from build123d import *

# Parameters (mm, degrees)
BOSS_EXTRUDE1_DEPTH = 5.7
SKETCH2_R           = 14.85
CUT_EXTRUDE1_DEPTH  = 6.7


with BuildPart() as part:
    # Sketch1 → Boss-Extrude1 (new body)
    with BuildSketch(Plane.XY):
        Polygon((-159.83650641, 166.052929421), (-154.13650641, 166.052929421), (-154.13650641, 115.252929421), (-160.286019508, 115.252929421), (-160.286019508, 50.952929421), (-154.13650641, 50.952929421), (-154.13650641, 0.152929421), (-159.83650641, 0.152929421), (-159.83650641, -24.847070579), (444.06349359, -24.847070579), (444.06349359, 0.899402865), (438.36349359, 0.899402865), (438.36349359, 51.699402865), (444.06349359, 51.699402865), (444.06349359, 77.821679421), (-159.83650641, 191.052929421), align=None)
    extrude(amount=BOSS_EXTRUDE1_DEPTH)

    # Sketch2 → Cut-Extrude1 (cut, through all)
    with BuildSketch(Plane.XY.offset(5.7)):
        with Locations((317.523696403, 24.846574105)):
            Circle(SKETCH2_R)
        Polygon((287.261228118, 47.129406511), (288.311706475, 52.731771656), (238.381855706, 62.093929643), (237.331377349, 56.491564498), align=None)
        Polygon((177.179115935, 67.770488147), (178.229594292, 73.372853292), (128.299743522, 82.735011279), (127.249265166, 77.132646134), align=None)
        Polygon((-92.56491366, 124.199043845), (-41.76491366, 114.673727458), (-42.83369916, 108.973727458), (-93.63369916, 118.499043845), align=None)
        Polygon((18.217631339, 103.376092915), (68.147482108, 94.013934928), (67.097003751, 88.411569783), (17.167152982, 97.77372777), align=None)
        with BuildLine():
            Line((-24.756085794, 42.151529897), (-24.756085794, 36.301350189))
            ThreePointArc((-24.756085794, 36.301350189), (-25.048979012, 35.594243408), (-25.756085794, 35.301350189))
            Line((-25.756085794, 35.301350189), (-125.756085794, 35.301350189))
            ThreePointArc((-125.756085794, 35.301350189), (-126.463192575, 35.594243408), (-126.756085794, 36.301350189))
            Line((-126.756085794, 36.301350189), (-126.756085794, 42.151529897))
            ThreePointArc((-126.756085794, 42.151529897), (-126.463192575, 42.858636678), (-125.756085794, 43.151529897))
            Line((-125.756085794, 43.151529897), (-25.756085794, 43.151529897))
            ThreePointArc((-25.756085794, 43.151529897), (-25.048979012, 42.858636678), (-24.756085794, 42.151529897))
        make_face()
        Polygon((348.312558617, 41.531771968), (347.252926688, 35.880589395), (398.052926688, 26.355273008), (399.112558617, 32.006455581), align=None)
        with BuildLine():
            Line((-25.756085794, 56.60407475), (-125.756085794, 56.60407475))
            ThreePointArc((-125.756085794, 56.60407475), (-126.463192575, 56.311181531), (-126.756085794, 55.60407475))
            Line((-126.756085794, 55.60407475), (-126.756085794, 49.753895042))
            ThreePointArc((-126.756085794, 49.753895042), (-126.463192575, 49.046788261), (-125.756085794, 48.753895042))
            Line((-125.756085794, 48.753895042), (-25.756085794, 48.753895042))
            ThreePointArc((-25.756085794, 48.753895042), (-25.048979012, 49.046788261), (-24.756085794, 49.753895042))
            Line((-24.756085794, 49.753895042), (-24.756085794, 55.60407475))
            ThreePointArc((-24.756085794, 55.60407475), (-25.048979012, 56.311181531), (-25.756085794, 56.60407475))
        make_face()
        with BuildLine():
            Line((-25.756085794, 29.698985049), (-125.756085794, 29.698985049))
            ThreePointArc((-125.756085794, 29.698985049), (-126.463192575, 29.40609183), (-126.756085794, 28.698985049))
            Line((-126.756085794, 28.698985049), (-126.756085794, 22.848805341))
            ThreePointArc((-126.756085794, 22.848805341), (-126.463192575, 22.14169856), (-125.756085794, 21.848805341))
            Line((-125.756085794, 21.848805341), (-25.756085794, 21.848805341))
            ThreePointArc((-25.756085794, 21.848805341), (-25.048979012, 22.14169856), (-24.756085794, 22.848805341))
            Line((-24.756085794, 22.848805341), (-24.756085794, 28.698985049))
            ThreePointArc((-24.756085794, 28.698985049), (-25.048979012, 29.40609183), (-25.756085794, 29.698985049))
        make_face()
    extrude(amount=-CUT_EXTRUDE1_DEPTH, mode=Mode.SUBTRACT)


solid = part.part
Could you check a few things on this model? Use its own coordinates, in mm. Give positions to 0.01 mm unless a question says otherwise; leave off trailing zeros. Loops run counter-clockwise (first coordinate to the right, second up) from the corner with the lowest first, then second, coordinate; pieces in that order, holes last. Notation, with made-up numbers: (-16, -1) -> (0, -1) arc R21 cw to (0, 14) -> close; hole circle Ø8 at (-33, 46.25). An arc over 180 degrees is marked (long way). Return JSON: item names as keys, results as strings.
Item 1: If we section it at D-D on z = 3.8: Count the separate pieces of the cut face and the enclosed holes in it, plus the area to 3 significant figures.
Geometry results:
{"separate pieces": "1", "enclosed holes": "9", "area": "90,800 mm²"}
Item 2: I'm going to push flat-ended pins straight in: pin 1 (1.5 mm diameter, centred on y = 126.5, z = 2, fed in from -X); pin 2 (3 mm diameter, centred on x = -98.5, z = 2.5, fed in from +Y); pin 3 (3 mm diameter, centred on y = 40, z = 2, fed in from +X). Where does each tip first touch, or does it pass through?
Geometry results:
{"pin 1": "stops at x = -154.14", "pin 2": "stops at y = 179.83", "pin 3": "stops at x = 438.36"}
Item 3: If we section it at C-C on x = 261: List the corners of the cut face in (y, z) for me.
Geometry results:
{"outline": "(-24.85, 0) -> (52.05, 0) -> (52.05, 5.7) -> (-24.85, 5.7) -> close; (57.85, 0) -> (112.15, 0) -> (112.15, 5.7) -> (57.85, 5.7) -> close"}
Item 4: I need wall thicknesses on L1, parallel to X at y = 26, z = 1.7; L2, parallel to X at y = -10, z = 4.6; L3, parallel to Y at x = 378, z = 0.4. Which ranges of each line are inside material? Lowest first, please. Write a range as from..to.
Geometry results:
{"L1": "x = -154.14..-126.76, -24.76..302.72, 332.33..438.36", "L2": "x = -159.84..444.06", "L3": "y = -24.85..30.12, 35.97..90.21"}
Item 5: If we section it at B-B on x = -77: List the corners of the cut face in (y, z) for me, plus the area to 3 significant figures.
Geometry results:
{"outline": "(-24.85, 0) -> (21.85, 0) -> (21.85, 5.7) -> (-24.85, 5.7) -> close; (29.7, 0) -> (35.3, 0) -> (35.3, 5.7) -> (29.7, 5.7) -> close; (43.15, 0) -> (48.75, 0) -> (48.75, 5.7) -> (43.15, 5.7) -> close; (56.6, 0) -> (115.38, 0) -> (115.38, 5.7) -> (56.6, 5.7) -> close; (121.28, 0) -> (175.52, 0) -> (175.52, 5.7) -> (121.28, 5.7) -> close", "area": "974 mm²"}
Item 6: If we section it at A-A on x = 25: List the corners of the cut face in (y, z) for me.
Geometry results:
{"outline": "(-24.85, 0) -> (96.31, 0) -> (96.31, 5.7) -> (-24.85, 5.7) -> close; (102.1, 0) -> (156.4, 0) -> (156.4, 5.7) -> (102.1, 5.7) -> close"}
